```python
from build123d import *

# Parameters (mm, degrees)
F1_DEPTH = 10
F2_R     = 2.25
F3_DEPTH = 25


with BuildPart() as f1:
    # F0 (on Top) → F1 (new body)
    with BuildSketch(Plane.XY):
        with BuildLine():
            ThreePointArc((-4.545297, 2.083333), (0.204825, 4.995803), (4.700586, 1.704257))
            ThreePointArc((4.700586, 1.704257), (4.814012, 1.556152), (4.991909, 1.5))
            Line((4.991909, 1.5), (23.835874, 1.5))
            ThreePointArc((23.835874, 1.5), (24.036696, 1.57388), (24.14176, 1.760291))
            ThreePointArc((24.14176, 1.760291), (34.729685, 10.996678), (45.758637, 2.291667))
            ThreePointArc((45.758637, 2.291667), (46.107542, 1.722718), (46.736695, 1.5))
            ThreePointArc((46.736695, 1.5), (47.513976, 1.870847), (47.714752, 2.708333))
            ThreePointArc((47.714752, 2.708333), (37.03088, 12.840386), (23.74167, 6.5))
            ThreePointArc((23.74167, 6.5), (23.009619, 5.767949), (22.009619, 5.5))
            Line((22.009619, 5.5), (4.974937, 5.5))
            ThreePointArc((4.974937, 5.5), (4.397587, 5.585146), (3.869396, 5.833333))
            ThreePointArc((3.869396, 5.833333), (-1.918794, 6.731882), (-6.363415, 2.916667))
            ThreePointArc((-6.363415, 2.916667), (-6.295981, 1.959938), (-5.454356, 1.5))
            ThreePointArc((-5.454356, 1.5), (-4.914294, 1.658375), (-4.545297, 2.083333))
        make_face()
    extrude(amount=F1_DEPTH)

    # F2 (on face) → F3 (cut)
    with BuildSketch(Plane.XZ.offset(-1.5)):
        with Locations((15, 5)):
            Circle(F2_R)
    extrude(amount=-F3_DEPTH, mode=Mode.SUBTRACT)


solid = f1.part
```
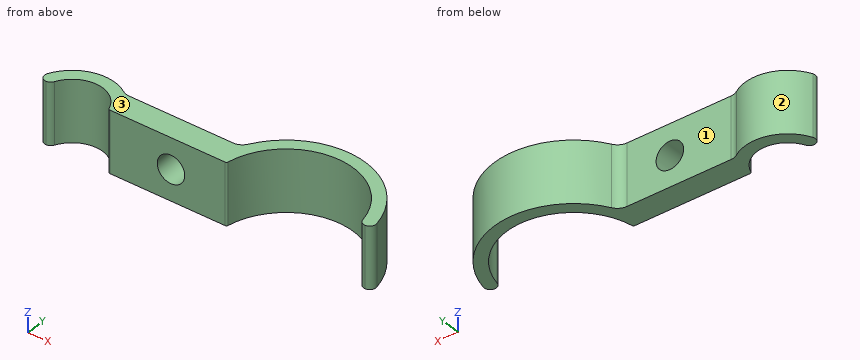
Could you check a few things on this model? Use its own coordinates, in mm. Face numbers are marked on the shaded views. Coordinates: 2 decimals unless noted, no trailing zeros. Loops run counter-clockwise (first coordinate to the right, second up) from the corner with the lowest first, then second, coordinate; pieces in that order, holes last.
1) Imagine slicing it at C-C (y = 8.75). List the corners of the cut face in (x, z) for me, and give its area (3 significant figures).
Reported:
outline: (25.39, 0) - (28.33, 0) - (28.33, 10) - (25.39, 10) - close; (41.67, 0) - (44.61, 0) - (44.61, 10) - (41.67, 10) - close
area: 59.0 mm2
2) Will these pins go through, and if not, where does the flat tip stop? pin 1 Ø1.5 at (x, z) = (32, 1.5) entering from -Y; pin 2 Ø5 at (y, z) = (9, 8) entering from +X; pin 3 Ø5 at (x, z) = (7.5, 2.5) entering from +Y.
Reported:
pin 1: stops at y = 10.34
pin 2: stops at x = 46.26
pin 3: stops at y = 5.5
3) Imagine slicing it at B-B (z = 5). List the corners of the cut face in (x, y) for me, and give its area (3 significant figures).
Reported:
outline: (-6.36, 2.92) arc R1 ccw to (-4.55, 2.08) arc R5 cw to (4.7, 1.7) arc R0.31 ccw to (4.99, 1.5) - (12.75, 1.5) - (12.75, 5.5) - (4.97, 5.5) arc R2 cw to (3.87, 5.83) arc R7 ccw to start; (17.25, 1.5) - (23.84, 1.5) arc R0.31 ccw to (24.14, 1.76) arc R11 cw to (45.76, 2.29) arc R1 ccw to (47.71, 2.71) arc R13 ccw to (23.74, 6.5) arc R2 cw to (22.01, 5.5) - (17.25, 5.5) - close
area: 149 mm2
4) Imagine slicing it at A-A (x = 15). List the corners of the cut face in (y, z) for me, and give its area (3 significant figures).
Reported:
outline: (1.5, 0) - (5.5, 0) - (5.5, 2.75) - (1.5, 2.75) - close; (1.5, 7.25) - (5.5, 7.25) - (5.5, 10) - (1.5, 10) - close
area: 22.0 mm2
5) Imagine slicing it at D-D (z = 8). List the corners of the cut face in (x, y) for me, and give its area (3 significant figures).
Reported:
outline: (-6.36, 2.92) arc R1 ccw to (-4.55, 2.08) arc R5 cw to (4.7, 1.7) arc R0.31 ccw to (4.99, 1.5) - (23.84, 1.5) arc R0.31 ccw to (24.14, 1.76) arc R11 cw to (45.76, 2.29) arc R1 ccw to (47.71, 2.71) arc R13 ccw to (23.74, 6.5) arc R2 cw to (22.01, 5.5) - (4.97, 5.5) arc R2 cw to (3.87, 5.83) arc R7 ccw to start
area: 167 mm2
6) Thinking about a two-plate mould opening in X: for the marked faces 1, 2 and 3, which applies, released by +X, released by -X, zero draft, split by the parting line, or undercut?
Reported:
face 1: undercut
face 2: undercut
face 3: zero draft
7) Please list where these lines run through material, in increasing order: line 1 along Z through (x, y) = (15, 3.45); line 2 along X through (y, z) = (5.75, 3); line 3 along Y through (x, z) = (19.5, 6.25).
Reported:
line 1: z = 0 to 2.75, 7.25 to 10
line 2: x = -3.99 to 4.01, 22.98 to 25.62, 44.38 to 46.66
line 3: y = 1.5 to 5.5
